Input: part model. Units: mm. Frame: model coordinates. A direction names the side the tool comes from. Give positions to 0.01 mm unless a question says otherwise; leave off trailing zeros. Write each loop counter-clockwise with the first axis right and the second up, starting at its lowest first coordinate (ties: lowest second). Pieces come first, ordered by that corner, then holes. Notation, with made-up numbers: (-31.75, 82) -> (-14.75, 82) arc R17 ccw to (-14.75, 109) -> close; hole circle Ø7 at (55.5, -35.75). An arc over 180 degrees is marked (long way). Return JSON: item names as keys, results as strings. Group by question number.
Item 1: Set-up query: faces 1 (the face through (0, 9, -2.5)), 2 (the face through (2.5, 9, 0)), 3 (the face through (2, 10, 2)), 4 (the face through (0, 9, 2.5)). Return all of +Z, -Z, +X, -X, +Y, -Y with unobstructed straight access to the full face (end or side cutting, diameter ignored); none if empty.
Item 2: Line query: line 1 (X direction, y = 9, z = -2.25); line 2 (Z direction, x = -4.5, y = 4.5); line 3 (Y direction, x = -2.5, z = -3.5). Output: solid intervals per line, ascending. Write a range as [from, to].
Item 3: Section A-A, the plane y = 18. Return loops of the section in (x, z), then the cut area to 3 significant figures.
Item 4: Pin query (flat end, axial travel): P1, Ø4, axis at x = -0.5, z = 3, coming from the +Y side; P2, Ø10, axis at y = -6, z = 6.5, coming from the -X side; P3, Ø1, axis at y = 9, z = 1, coming from the -X side; P4, Ø1.6, axis at x = -0.5, y = 9, coming from the -Z side. Return the tip coordinate at first contact, or that it passes through.
from build123d import *

# Parameters (mm, degrees)
SKETCH2_W           = 5
SKETCH2_H           = 5
BOSS_EXTRUDE1_DEPTH = 2
SKETCH3_R           = 2.5
BOSS_EXTRUDE2_DEPTH = 14


with BuildPart() as part:
    # Sketch1 → Revolve1 (revolve)
    with BuildSketch(Plane.XY):
        with BuildLine():
            Line((0, 8), (4.95, 8))
            add(Edge.make_bspline(
                [(0, -10), (24.75, -10), (4.95, 8)],
                knots=[3.141592654, 3.141592654, 3.141592654, 5.639684198, 5.639684198, 5.639684198], degree=2, weights=[1, 0.316227766, 1]))
            Line((0, -10), (0, 8))
        make_face()
    revolve(axis=Axis((0, 8, 0), (0, -1, 0)))

    # Sketch2 → Boss-Extrude1 (add)
    with BuildSketch(Plane(origin=(0, 8, 0), x_dir=(1, 0, 0), z_dir=(0, 1, 0))):
        Rectangle(SKETCH2_W, SKETCH2_H)
    extrude(amount=BOSS_EXTRUDE1_DEPTH)

    # Sketch3 → Boss-Extrude2 (add)
    with BuildSketch(Plane(origin=(0, 10, 0), x_dir=(1, 0, 0), z_dir=(0, 1, 0))):
        with Locations(Location((0, 0, 0), (0, 0, 180))):
            Circle(SKETCH3_R)
    extrude(amount=BOSS_EXTRUDE2_DEPTH)

    # Sketch4 → Revolve3 (revolve)
    with BuildSketch(Plane.XY, mode=Mode.PRIVATE) as revolve3_sk:
        with BuildLine():
            Line((-0.001464112, 6), (6.708203932, 6))
            ThreePointArc((6.708203932, 6), (8.215539475, -3.674902875), (-0.001464112, -8.999999881))
            Line((-0.001464112, -8.999999881), (-0.001464112, 6))
        make_face()
    revolve(revolve3_sk.sketch.rotate(Axis((-0.001464112, 6, 0), (0, -1, 0)), 180), axis=Axis((-0.001464112, 6, 0), (0, -1, 0)))


solid = part.part
Answer below:
{
 "1": {"face 1": "-Z, +X, -X, +Y", "face 2": "+Z, -Z, +X, +Y", "face 3": "+Z, +X, +Y", "face 4": "+Z, +X, -X, +Y"},
 "2": {"line 1": "x = [-2.5, 2.5]", "line 2": "z = [-6.37, 6.37]", "line 3": "y = [-8.53, 8]"},
 "3": {"outline": "circle Ø5 at (0, 0)", "area": "19.6 mm2"},
 "4": {"P1": "stops at y = 24", "P2": "stops at x = -8.14", "P3": "stops at x = -2.5", "P4": "stops at z = -2.5"}
}
